Model file for the job. Use its own axes, mm. A direction names the side the tool comes from. Coordinates: 2 decimals unless noted, no trailing zeros. Write each loop counter-clockwise with the first axis right and the second up, starting at its lowest first coordinate (ties: lowest second). Pieces come first, ordered by that corner, then holes. Notation, with made-up numbers: M -25,-11.5 L -10,-11.5 A17 cw -10,-5.5 Z; hole C 49.5,76.25 d11. An arc over 180 degrees is marked long. Put each result on its own line as item: value. Start each with the question number.
Q1. Cut at C-C (z = 8.5). Give the number of separate pieces and of enclosed holes in the cut face, then the cut area to 3 significant figures.
Q2. Which spindle directions (+Z, -Z, +X, -X, +Y, -Y) get a long thin tool onto all of the face, cutting with end or side? Do faces 4 (the cylindrical face through (-7.357, 1.244, 11.753)), 5 (the cylindrical face through (13, 0, 1)), 6 (the cylindrical face through (5.22, -7.47, 5.42)). Say none if no direction does.
Q3. Cut at B-B (x = -2). Write the cut outline in (y, z).
Q4. Drop flat-ended pins along their axis: pin 1 (2 mm diameter, centred on x = -8.5, z = 14.5, fed in from +Y); pin 2 (6 mm diameter, centred on x = 9.5, y = -6, fed in from +Z); pin 3 (4 mm diameter, centred on x = -2, z = 17, fed in from +Y). Give the stop position or say it passes through.
Q5. Cut at A-A (x = -7). Write the cut outline in (y, z), then the cut area to 3 significant figures.
Q6. Drill centre lines: line 1 along X through (y, z) = (2.5, 15); line 2 along Y through (x, z) = (4.95, 8.5); line 3 along X through (y, z) = (-9.5, 15). Where is each one in solid material? Low to high.
Q7. Pull direction X, two halves, no side cores. Call faces 1 (the flat face through (0, -12, 30)), 2 (the cylindrical face through (14.43, 3.535, 13.883)), 3 (the flat face through (6, -1.75, 16)): pulls with the +X half, pulls with the -X half, needs draft (parallel to the pull), parting line crosses it, or undercut.
```python
from build123d import *

# Parameters (mm, degrees)
SKETCH1_W              = 30
SKETCH1_H              = 27.5
EXTRUDE1_DEPTH         = 30
EXTRUDE3_DEPTH         = 45.598906937
SKETCH7_R              = 1.25
CUT_EXTRUDE_1045_DEPTH = 11
SKETCH8_R              = 3.25
EXTRUDE8_DEPTH         = 15.5
EXTRUDE9_DEPTH         = 44.373378932
EXTRUDE9_DEPTH_BACK    = 44.373378932
SKETCH9_R              = 1.5
FILLET1_R              = 5
FILLET3_R              = 2


with BuildPart() as part:
    # Sketch1 → Extrude1 (new body)
    with BuildSketch(Plane.XY):
        Rectangle(SKETCH1_W, SKETCH1_H)
    extrude(amount=EXTRUDE1_DEPTH)

    # Sketch3 → Extrude3 (cut, through all)
    with BuildSketch(Plane(origin=(15, 0, 0), x_dir=(0, 0, -1), z_dir=(1, 0, 0))):
        Polygon((-30, -6.75), (-30, 13.75), (0, 13.75), align=None)
    extrude(amount=-EXTRUDE3_DEPTH, mode=Mode.SUBTRACT)

    # Sketch7 → Cut-Extrude 1045 (cut)
    with BuildSketch(Plane(origin=(0, 0, 0), x_dir=(-1, 0, 0), z_dir=(0, 0, -1))):
        with Locations((-4.95, 3.65)):
            Circle(SKETCH7_R)
        with Locations((4.95, 3.65)):
            Circle(SKETCH7_R)
        with Locations((4.95, -6.25)):
            Circle(SKETCH7_R)
        with Locations((-4.95, -6.25)):
            Circle(SKETCH7_R)
    extrude(amount=-CUT_EXTRUDE_1045_DEPTH, mode=Mode.SUBTRACT)

    # Sketch8 → Extrude8 (cut)
    with BuildSketch(Plane(origin=(0, 13.75, 0), x_dir=(1, 0, 0), z_dir=(0, 1, 0))):
        with Locations(Location((-7.5, -15, 0), (0, 0, 270))):
            Circle(SKETCH8_R)
        with Locations(Location((7.5, -15, 0), (0, 0, 270))):
            Circle(SKETCH8_R)
    extrude(amount=-EXTRUDE8_DEPTH, mode=Mode.SUBTRACT)

    # Sketch9 → Extrude9 (cut, two sides: drawn at the far end of the back side and taken through both)
    with BuildSketch(Plane(origin=(0, 13.75, 0), x_dir=(1, 0, 0), z_dir=(0, 1, 0)).offset(-EXTRUDE9_DEPTH_BACK)):
        with Locations(Location((-7.5, -15, 0), (0, 0, 270))):
            Circle(SKETCH9_R)
        with Locations(Location((7.5, -15, 0), (0, 0, 270))):
            Circle(SKETCH9_R)
    extrude(amount=EXTRUDE9_DEPTH + EXTRUDE9_DEPTH_BACK, mode=Mode.SUBTRACT)

    # Fillet1
    fillet1_edges = [part.edges().sort_by_distance(p)[0] for p in [
        (0, -6.75, 30),
        (15, 0, 0),
        (-15, 0, 0),
    ]]
    fillet(fillet1_edges, radius=FILLET1_R)

    # Fillet3
    # the kernel refuses this fillet: 2 mm, written as the material it takes off along each edge
    with BuildSketch(Plane(origin=(15, -18.75, 30), x_dir=(-1, 0, 0), z_dir=(0, 1, 0))) as fillet3_piece_1:
        with BuildLine():
            CenterArc((FILLET3_R, -FILLET3_R), FILLET3_R, 90, 90)
            Line((0, -FILLET3_R), (0, 0))
            Line((0, 0), (FILLET3_R, 0))
        make_face()
    extrude(amount=9.360792567, mode=Mode.SUBTRACT)
    with BuildSketch(Plane(origin=(-15, -9.389207433, 30), x_dir=(0, 0, -1), z_dir=(0, -1, 0))) as fillet3_piece_2:
        with BuildLine():
            CenterArc((FILLET3_R, FILLET3_R), FILLET3_R, 180, 90)
            Line((0, FILLET3_R), (0, 0))
            Line((0, 0), (FILLET3_R, 0))
        make_face()
    extrude(amount=9.360792567, mode=Mode.SUBTRACT)
    with BuildSketch(Plane(origin=(-15, 13.154285858, 0.871776792), x_dir=(0, -0.8256446415008141, -0.5641905050255563), z_dir=(0, -0.5641905050255562, 0.8256446415008141))) as fillet3_piece_3:
        with BuildLine():
            CenterArc((FILLET3_R, FILLET3_R), FILLET3_R, 180, 90)
            Line((0, FILLET3_R), (0, 0))
            Line((0, 0), (FILLET3_R, 0))
        make_face()
    extrude(amount=32.640163065, mode=Mode.SUBTRACT)
    with BuildSketch(Plane(origin=(15, 13.154285858, 0.871776792), x_dir=(0, -0.8256446415008141, -0.5641905050255563), z_dir=(0, -0.5641905050255562, 0.8256446415008141))) as fillet3_piece_4:
        with BuildLine():
            CenterArc((FILLET3_R, -FILLET3_R), FILLET3_R, 90, 90)
            Line((0, -FILLET3_R), (0, 0))
            Line((0, 0), (FILLET3_R, 0))
        make_face()
    extrude(amount=32.640163065, mode=Mode.SUBTRACT)
    with BuildSketch(Plane(origin=(15, -9.389207433, 25), x_dir=(0, 0, 1), z_dir=(0, -1, 0))) as fillet3_piece_5:
        with BuildLine():
            CenterArc((5 - FILLET3_R, FILLET3_R), FILLET3_R, 270, 90)
            Line((5, FILLET3_R), (5, 0))
            Line((5, 0), (5 - FILLET3_R, 0))
        make_face()
    revolve(axis=Axis((15, -9.389207433, 25), (-1, 0, 0)), revolution_arc=55.6539026, mode=Mode.SUBTRACT)
    with BuildSketch(Plane(origin=(-15, -9.389207433, 25), x_dir=(0, 0, 1), z_dir=(0, -1, 0))) as fillet3_piece_6:
        with BuildLine():
            CenterArc((5 - FILLET3_R, -FILLET3_R), FILLET3_R, 0, 90)
            Line((5, -FILLET3_R), (5, 0))
            Line((5, 0), (5 - FILLET3_R, 0))
        make_face()
    revolve(axis=Axis((-15, -9.389207433, 25), (-1, 0, 0)), revolution_arc=55.6539026, mode=Mode.SUBTRACT)


solid = part.part
```
Computed values:
1. separate pieces: 1
1. enclosed holes: 4
1. area: 629 mm2
2. face 4: +Y
2. face 5: -Z, +X, +Y, -Y
2. face 6: -Z
3. outline: M -13.75,0 L 13.75,0 L -5.26,27.82 A5 ccw -9.39,30 L -13.75,30 Z
4. pin 1: y = -1.75
4. pin 2: z = 29.98
4. pin 3: y = 3.5
5. outline: M -13.75,0 L 13.75,0 L 5.69,11.79 L -1.75,11.79 L -1.75,13.59 L -13.75,13.59 Z; M -13.75,16.41 L -1.75,16.41 L -1.75,18.21 L 1.31,18.21 L -5.26,27.82 A5 ccw -9.39,30 L -13.75,30 Z
5. area: 449 mm2
6. line 1: -14.62 to -10.75, -4.25 to 4.25, 10.75 to 14.62
6. line 2: -13.75 to -7.5, -5 to 2.4, 4.9 to 7.94
6. line 3: -15 to -9, -6 to 6, 9 to 15
7. face 1: needs draft
7. face 2: pulls with the +X half
7. face 3: undercut
